from build123d import *

# Parameters (mm, degrees)
CROQUIS1_R                   = 2.7
CROQUIS1_R_2                 = 20
SALIENTE_EXTRUIR1_DEPTH      = 6
SALIENTE_EXTRUIR2_DEPTH      = 56
SALIENTE_EXTRUIR2_DEPTH_BACK = 6
CROQUIS3_W                   = 20.2
CROQUIS3_H                   = 20.4
CORTAR_EXTRUIR1_DEPTH        = 110.967852121


with BuildPart() as part:
    # Croquis1 → Saliente-Extruir1 (new body)
    with BuildSketch(Plane.XY):
        with BuildLine():
            Line((-8, -50.14), (-8, 3))
            ThreePointArc((-8, 3), (-6.535533906, 6.535533906), (-3, 8))
            Line((-3, 8), (50.14, 8))
            ThreePointArc((50.14, 8), (53.675533906, 6.535533906), (55.14, 3))
            Line((55.14, 3), (55.14, -50.14))
            ThreePointArc((55.14, -50.14), (53.675533906, -53.675533906), (50.14, -55.14))
            Line((50.14, -55.14), (-3, -55.14))
            ThreePointArc((-3, -55.14), (-6.535533906, -53.675533906), (-8, -50.14))
        make_face()
        Circle(CROQUIS1_R, mode=Mode.SUBTRACT)
        with Locations((47.14, 0)):
            Circle(CROQUIS1_R, mode=Mode.SUBTRACT)
        with Locations((47.14, -47.14)):
            Circle(CROQUIS1_R, mode=Mode.SUBTRACT)
        with Locations((0, -47.14)):
            Circle(CROQUIS1_R, mode=Mode.SUBTRACT)
        with Locations((23.57, -23.57)):
            Circle(CROQUIS1_R_2, mode=Mode.SUBTRACT)
    extrude(amount=SALIENTE_EXTRUIR1_DEPTH)

    # Croquis2 → Saliente-Extruir2 (add, two sides: drawn at the far end of the back side and taken through both)
    with BuildSketch(Plane.XY.offset(6).offset(-SALIENTE_EXTRUIR2_DEPTH_BACK)):
        with BuildLine():
            ThreePointArc((-3, -55.14), (-6.535533906, -53.675533906), (-8, -50.14))
            Line((-8, -50.14), (-8, -67.17))
            ThreePointArc((-8, -67.17), (-6.535533906, -70.705533906), (-3, -72.17))
            Line((-3, -72.17), (13.47, -72.17))
            Line((13.47, -72.17), (13.47, -55.14))
            Line((13.47, -55.14), (-3, -55.14))
        make_face()
        with BuildLine():
            Line((55.14, -67.17), (55.14, -50.14))
            ThreePointArc((55.14, -50.14), (53.675533906, -53.675533906), (50.14, -55.14))
            Line((50.14, -55.14), (33.67, -55.14))
            Line((33.67, -55.14), (33.67, -72.17))
            Line((33.67, -72.17), (50.14, -72.17))
            ThreePointArc((50.14, -72.17), (53.675533906, -70.705533906), (55.14, -67.17))
        make_face()
        with BuildLine():
            Line((13.47, -51.77), (-4.63, -51.77))
            Line((-4.63, -51.77), (-4.63, -50.14))
            Line((-4.63, -50.14), (-8, -50.14))
            ThreePointArc((-8, -50.14), (-6.535533906, -53.675533906), (-3, -55.14))
            Line((-3, -55.14), (13.47, -55.14))
            Line((13.47, -55.14), (13.47, -51.77))
        make_face()
        with BuildLine():
            Line((55.14, -50.14), (51.77, -50.14))
            Line((51.77, -50.14), (51.77, -51.77))
            Line((51.77, -51.77), (33.67, -51.77))
            Line((33.67, -51.77), (33.67, -55.14))
            Line((33.67, -55.14), (50.14, -55.14))
            ThreePointArc((50.14, -55.14), (53.675533906, -53.675533906), (55.14, -50.14))
        make_face()
    extrude(amount=SALIENTE_EXTRUIR2_DEPTH + SALIENTE_EXTRUIR2_DEPTH_BACK)

    # Croquis3 → Cortar-Extruir1 (cut, through all)
    with BuildSketch(Plane.XY.offset(62)):
        with Locations((23.57, -61.97)):
            Rectangle(CROQUIS3_W, CROQUIS3_H)
    extrude(amount=-CORTAR_EXTRUIR1_DEPTH, mode=Mode.SUBTRACT)


solid = part.part
Part model, mm, in its own coordinate system. A direction names the side the tool comes from. Coordinates: 2 decimals unless noted, no trailing zeros. Loops run counter-clockwise (first coordinate to the right, second up) from the corner with the lowest first, then second, coordinate; pieces in that order, holes last. Notation, with made-up numbers: (-3, 20.25) -> (45, 20.25) arc R27 ccw to (45, 37.25) -> close; hole circle Ø8 at (69.5, 26). An arc over 180 degrees is marked (long way). Use a Markdown table: item, result. Add a question column.
Item 1: Pull direction Y, two halves, no side cores. Call faces 1 (the cylindrical face through (-0.351, -44.463, 2.958)), 2 (the flat face through (5, -51.77, 34)), 3 (the flat face through (-8, -53, 22)): +Y half, -Y half, draft (parallel to the pull), parting line (faces both ways), or undercut.
Item 2: Band-saw the part on B-B on y = -65.5. Write the cut outline in (x, z).
Item 3: Band-saw the part on A-A on x = 47.14. Write the cut outline in (y, z).
Item 4: Which spindle directions (+Z, -Z, +X, -X, +Y, -Y) get a long thin tool onto all of the face, cutting with end or side? Do faces 4 (the flat face through (23, -51.77, 3)), 5 (the flat face through (43, -51.77, 34)), 6 (the flat face through (-6, -50.14, 34)). Say none if no direction does.
Item 5: Band-saw the part on D-D on y = 0. Write the cut outline in (x, z).
Item 6: Probe probe 1 along X at (y, z) = (-47, 3); probe 2 along Y at (x, z) = (0, 1.55); probe 3 along X at (y, z) = (-61, 30.5). List the from-to ranges inside material, lowest first.
Item 7: Band-saw the part on C-C on z = 38.5. Write the cut outline in (x, y), plus the area to 3 significant figures.
Item 8: Flat gauge pins, fed straight in: P1, Ø2, axis at y = -49, z = 18, coming from the +X side; P2, Ø1.7, axis at x = 53, z = 25.5, coming from the +Y side; P3, Ø14.5, axis at x = 4, z = 32, coming from the +Y side; P4, Ø5, axis at x = 25, z = 3.5, coming from the -Y side. Where does each tip first touch, or does it go through?
Geometry says:
| question | item | result |
|---|---|---|
| 1 | face 1 | undercut |
| 1 | face 2 | +Y half |
| 1 | face 3 | draft |
| 2 | outline | (-8, 0) -> (13.47, 0) -> (13.47, 62) -> (-8, 62) -> close; (33.67, 0) -> (55.14, 0) -> (55.14, 62) -> (33.67, 62) -> close |
| 3 | outline | (-72.17, 0) -> (-49.84, 0) -> (-49.84, 6) -> (-51.77, 6) -> (-51.77, 62) -> (-72.17, 62) -> close; (-44.44, 0) -> (-2.7, 0) -> (-2.7, 6) -> (-44.44, 6) -> close; (2.7, 0) -> (8, 0) -> (8, 6) -> (2.7, 6) -> close |
| 4 | face 4 | +Z, -Z, -Y |
| 4 | face 5 | +Z, +Y |
| 4 | face 6 | +Z, +X, -X, +Y |
| 5 | outline | (-8, 0) -> (-2.7, 0) -> (-2.7, 6) -> (-8, 6) -> close; (2.7, 0) -> (44.44, 0) -> (44.44, 6) -> (2.7, 6) -> close; (49.84, 0) -> (55.14, 0) -> (55.14, 6) -> (49.84, 6) -> close |
| 6 | probe 1 | -8 to -2.7, 2.7 to 44.44, 49.84 to 55.14 |
| 6 | probe 2 | -72.17 to -49.84, -44.44 to -2.7, 2.7 to 8 |
| 6 | probe 3 | -8 to 13.47, 33.67 to 55.14 |
| 7 | outline | (-8, -67.17) arc R5 ccw to (-3, -72.17) -> (13.47, -72.17) -> (13.47, -51.77) -> (-4.63, -51.77) -> (-4.63, -50.14) -> (-8, -50.14) -> close; (33.67, -72.17) -> (50.14, -72.17) arc R5 ccw to (55.14, -67.17) -> (55.14, -50.14) -> (51.77, -50.14) -> (51.77, -51.77) -> (33.67, -51.77) -> close |
| 7 | area | 876 mm² |
| 8 | P1 | through |
| 8 | P2 | y = -50.14 |
| 8 | P3 | y = -51.77 |
| 8 | P4 | y = -51.77 |
